Model file for the job. Use its own axes, mm. Coordinates: 2 decimals unless noted, no trailing zeros. Order: outer loops, then holes, each group sorted by start corner. A loop starts at its lowest first (then second) coordinate and runs counter-clockwise, first axis right, second up. Notation, with made-up numbers: M 73,10.5 L 110,10.5 A32 ccw 110,36.5 Z; hole C 85,11.5 d4. An arc over 180 degrees is marked long. Return JSON: item names as keys, results as strings.
```python
from build123d import *

# Parameters (mm, degrees)
SKETCH1_R                 = 4.7625
BOSS_EXTRUDE1_DEPTH       = 11.1125
SKETCH2_W                 = 8.255
SKETCH2_H                 = 9.525
CUT_EXTRUDE1_DEPTH        = 0.508
F_4_40_TAPPED_HOLE1_D     = 2.2606
F_4_40_TAPPED_HOLE1_DEPTH = 3.81
F_4_40_TAPPED_HOLE1_TIP   = 0.679152758
CHAMFER1_SIZE             = 0.254


with BuildPart() as part:
    # Sketch1 → Boss-Extrude1 (new body, symmetric)
    with BuildSketch(Plane(origin=(0, 0, 0), x_dir=(0, 0, -1), z_dir=(1, 0, 0))):
        Circle(SKETCH1_R)
    extrude(amount=BOSS_EXTRUDE1_DEPTH, both=True)

    # Sketch2 → Cut-Extrude1 (cut)
    with BuildSketch(Plane(origin=(0, 0, -4.7625), x_dir=(-1, 0, 0), z_dir=(0, 0, -1))):
        Rectangle(SKETCH2_W, SKETCH2_H)
    extrude(amount=-CUT_EXTRUDE1_DEPTH, mode=Mode.SUBTRACT)

    # #4-40 Tapped Hole1
    with Locations(Plane(origin=(0, 0, -4.2545), x_dir=(-1, 0, 0), z_dir=(0, 0, -1))):
        with Locations((0, 0)):
            Hole(F_4_40_TAPPED_HOLE1_D / 2, depth=F_4_40_TAPPED_HOLE1_DEPTH)
            with Locations((0, 0, -(F_4_40_TAPPED_HOLE1_DEPTH + F_4_40_TAPPED_HOLE1_TIP / 2))):  # 118° drill point
                Cone(0, F_4_40_TAPPED_HOLE1_D / 2, F_4_40_TAPPED_HOLE1_TIP, mode=Mode.SUBTRACT)

    # Chamfer1
    chamfer1_edges = [part.edges().sort_by_distance(p)[0] for p in [
        (-11.1125, 0, 4.7625),
        (11.1125, 0, 4.7625),
    ]]
    chamfer(chamfer1_edges, length=CHAMFER1_SIZE)


solid = part.part
```
Item 1: Saw through at B-B (x = -9.25). Write the cut outline in (y, z) (1 decimal), and give its area (3 significant figures).
Check result:
{"outline": "C 0,0 d9.5", "area": "71.3 mm2"}
Item 2: Pull direction X, two halves, no side cores. Call faces 1 (the flat face through (-11.112, 0, 0)), 2 (the flat face through (11.112, 0, 0)), 3 (the flat face through (-1, 1, -4.254)), 4 (the cylindrical face through (-0.245, -1.103, -2.323)): +X half, -X half, draft (parallel to the pull), parting line (faces both ways), or undercut.
Check result:
{"face 1": "-X half", "face 2": "+X half", "face 3": "undercut", "face 4": "undercut"}
Item 3: Wall check: line 1 (X direction, y = 0, z = -2.8); line 2 (Y direction, x = 0, z = -1.55); line 3 (Y direction, x = 1, z = -3.5). Give the ranges that are in metal, low to high.
Check result:
{"line 1": "x = -11.11 to -1.13, 1.13 to 11.11", "line 2": "y = -4.5 to -1.13, 1.13 to 4.5", "line 3": "y = -3.23 to -0.53, 0.53 to 3.23"}
Item 4: Drop flat-ended pins along their axis: pin 1 Ø1 at (x, z) = (3.5, -3) entering from -Y; pin 2 Ø3.5 at (x, y) = (0.5, -0.5) entering from -Z. Give the stop position or say it passes through.
Check result:
{"pin 1": "stops at y = -4.05", "pin 2": "stops at z = -4.25"}
Item 5: Saw through at A-A (x = 3). Write the cut outline in (y, z) (1 decimal), and give its area (3 significant figures).
Check result:
{"outline": "M -2.1,-4.3 L 2.1,-4.3 A4.8 ccw long Z", "area": "69.8 mm2"}
